from build123d import *

# Parameters (mm, degrees)
SKETCH1_R           = 6
BOSS_EXTRUDE1_DEPTH = 6.35
SKETCH2_W           = 6.35
SKETCH2_H           = 38.1
SKETCH2_W_2         = 31.75
SKETCH2_H_2         = 6.35
MOTORMOUNT_DEPTH    = 38.1
SKETCH4_W           = 6.35
SKETCH4_H           = 25.4
WHEELMOUNTS_DEPTH   = 38.1
FILLET1_R           = 6.35
BOSS_EXTRUDE4_START = -2.54
SKETCH5_R           = 6
SKETCH5_R_2         = 4.5
BOSS_EXTRUDE4_DEPTH = 2.54
SKETCH6_R           = 6
CUT_EXTRUDE2_DEPTH  = 83.947
FILLET2_R           = 6.35


with BuildPart() as part:
    # Sketch1 → Boss-Extrude1 (new body)
    with BuildSketch(Plane(origin=(0, 0, 0), x_dir=(1, 0, 0), z_dir=(0, 1, 0))):
        with BuildLine():
            Line((50.8, 0), (50.8, -28.575))
            Line((50.8, -28.575), (39.852082176, -33.3375))
            ThreePointArc((39.852082176, -33.3375), (33.608374366, -42.8625), (39.852082176, -52.3875))
            Line((39.852082176, -52.3875), (50.8, -57.15))
            Line((50.8, -57.15), (82.55, -57.15))
            Line((82.55, -57.15), (93.497917824, -52.3875))
            ThreePointArc((93.497917824, -52.3875), (99.741625634, -42.8625), (93.497917824, -33.3375))
            Line((93.497917824, -33.3375), (82.55, -28.575))
            Line((82.55, -28.575), (82.55, 0))
            Line((82.55, 0), (133.35, 0))
            Line((133.35, 0), (133.35, 95.25))
            Line((133.35, 95.25), (104.775, 95.25))
            Line((104.775, 95.25), (104.775, 142.875))
            Line((104.775, 142.875), (28.575, 142.875))
            Line((28.575, 142.875), (28.575, 95.25))
            Line((28.575, 95.25), (0, 95.25))
            Line((0, 95.25), (0, 0))
            Line((0, 0), (50.8, 0))
        make_face()
        with Locations(Location((89.354407321, -42.8625, 0), (0, 0, 270))):
            Circle(SKETCH1_R, mode=Mode.SUBTRACT)
        with Locations(Location((43.995592679, -42.8625, 0), (0, 0, 90))):
            Circle(SKETCH1_R, mode=Mode.SUBTRACT)
    extrude(amount=BOSS_EXTRUDE1_DEPTH)

    # Sketch2 → MotorMount (add)
    with BuildSketch(Plane(origin=(0, 6.35, 0), x_dir=(1, 0, 0), z_dir=(0, 1, 0))):
        with Locations((130.175, 76.2)):
            Rectangle(SKETCH2_W, SKETCH2_H)
        with Locations((3.175, 76.2)):
            Rectangle(SKETCH2_W, SKETCH2_H)
        with Locations((15.875, 3.175)):
            Rectangle(SKETCH2_W_2, SKETCH2_H_2)
        with Locations((117.475, 3.175)):
            Rectangle(SKETCH2_W_2, SKETCH2_H_2)
    extrude(amount=MOTORMOUNT_DEPTH)

    # Sketch4 → WheelMounts (add)
    with BuildSketch(Plane(origin=(0, 6.35, 0), x_dir=(1, 0, 0), z_dir=(0, 1, 0))):
        with Locations((101.6, 130.175)):
            Rectangle(SKETCH4_W, SKETCH4_H)
        with Locations((31.75, 130.175)):
            Rectangle(SKETCH4_W, SKETCH4_H)
    extrude(amount=WHEELMOUNTS_DEPTH)

    # Fillet1
    fillet1_edges = [part.edges().sort_by_distance(p)[0] for p in [
        (82.55, 3.175, 0),
        (50.8, 3.175, 0),
    ]]
    fillet(fillet1_edges, radius=FILLET1_R)

    # Sketch5 → Boss-Extrude4 (add)
    # profile 1 of 2: a face of its own
    with BuildSketch(Plane(origin=(0, 6.35, 0), x_dir=(1, 0, 0), z_dir=(0, 1, 0)).offset(BOSS_EXTRUDE4_START)):
        with Locations(Location((43.995592679, -42.8625, 0), (0, 0, 90))):
            Circle(SKETCH5_R)
        with Locations(Location((43.995592679, -42.8625, 0), (0, 0, 270))):
            Circle(SKETCH5_R_2, mode=Mode.SUBTRACT)
    # profile 2 of 2: a face of its own
    with BuildSketch(Plane(origin=(0, 6.35, 0), x_dir=(1, 0, 0), z_dir=(0, 1, 0)).offset(BOSS_EXTRUDE4_START)):
        with Locations(Location((89.354407321, -42.8625, 0), (0, 0, 270))):
            Circle(SKETCH5_R)
        with Locations(Location((89.354407321, -42.8625, 0), (0, 0, 270))):
            Circle(SKETCH5_R_2, mode=Mode.SUBTRACT)
    extrude(amount=BOSS_EXTRUDE4_DEPTH)

    # Sketch6 → Cut-Extrude2 (cut)
    with BuildSketch(Plane(origin=(104.775, 0, 0), x_dir=(0, 0, -1), z_dir=(1, 0, 0))):
        with Locations((132.715, 12.35)):
            Circle(SKETCH6_R)
    extrude(amount=-CUT_EXTRUDE2_DEPTH, mode=Mode.SUBTRACT)

    # Fillet2
    fillet2_edges = [part.edges().sort_by_distance(p)[0] for p in [
        (28.575, 3.175, -95.25),
        (104.775, 3.175, -95.25),
    ]]
    fillet(fillet2_edges, radius=FILLET2_R)


solid = part.part
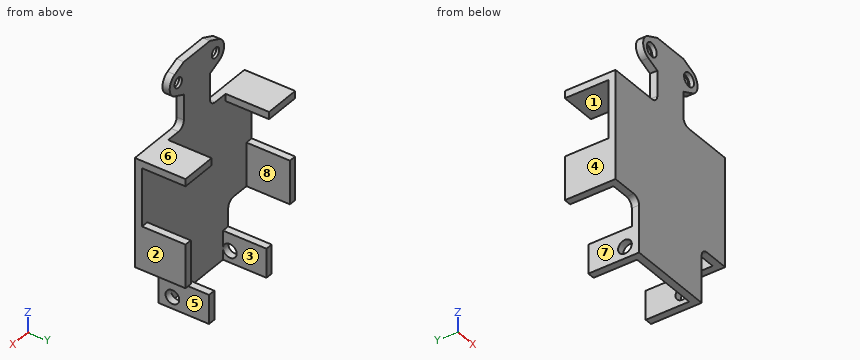
Geometry check sheet. Reference: the model listing, model coordinates, mm. Face numbers are marked on the shaded views. A direction names the side the tool comes from. Coordinates: 2 decimals unless noted, no trailing zeros. Loops run counter-clockwise (first coordinate to the right, second up) from the corner with the lowest first, then second, coordinate; pieces in that order, holes last. Notation, with made-up numbers: (-3.75, 88) - (16.25, 88) arc R19 cw to (16.25, 112) - close; hole circle Ø5 at (51.25, 78.5). An arc over 180 degrees is marked (long way). Use one line per item in the form item = value. Start each with the question number.
Item 1: Gauge pin test, flat ends, axial feed: pin 1 (6 mm diameter, centred on y = 25, z = -79, fed in from -X); pin 2 (13.5 mm diameter, centred on x = 113, y = 20, fed in from +Z); pin 3 (11 mm diameter, centred on y = 12.35, z = -132.715, fed in from -X); pin 4 (6 mm diameter, centred on x = 104, z = -29.5, fed in from +Y). Record the tip position at first contact, or that the pin passes through.
Item 2: Thickness scan on probe 1 along Z at (x, y) = (102, 12) (3 decimals); probe 2 along Z at (x, y) = (33, 12) (3 decimals); probe 3 along X at (y, z) = (26, -68). Record the ranges inside material, lowest first.
Item 3: Section check C-C, the plane z = -124. Enter the section's corners in (x, y) (3 decimals).
Item 4: Section check A-A, the plane y = 37. Enter the section's corners in (x, z) (3 decimals), and give its area (3 significant figures).
Item 5: Tool access check on the marked faces 1, 2, 3, 4 and 5. Record the directions out of +Z, -Z, +X, -X, +Y, -Y that give a thin tool (end or side, any length) a straight path to the whole face; none if there is none.
Item 6: Section check B-B, the plane y = 12.35. Give the number of separate pieces and of enclosed holes in the cut face, and give its area (3 significant figures).
Item 7: Section check D-D, the plane x = 15. Enter the section's corners in (y, z).
Item 8: Mould release check, pull along X, two halves, no side actions. Record for the marked faces 6, 7 and 8: +X half, -X half, draft (parallel to the pull), parting line (faces both ways), or undercut.
Computed:
q1.pin_1 = 0
q1.pin_2 = 0
q1.pin_3 = through
q1.pin_4 = 6.35
q2.probe_1 = -142.875 to -138.705, -126.725 to -117.475, -6.35 to 0
q2.probe_2 = -142.875 to -138.705, -126.725 to -117.475
q2.probe_3 = 0 to 6.35, 127 to 133.35
q3.outline = (28.575, 0) - (104.775, 0) - (104.775, 44.45) - (98.425, 44.45) - (98.425, 6.35) - (34.925, 6.35) - (34.925, 44.45) - (28.575, 44.45) - close
q4.outline = (0, -95.25) - (6.35, -95.25) - (6.35, -57.15) - (0, -57.15) - close; (0, -6.35) - (31.75, -6.35) - (31.75, 0) - (0, 0) - close; (28.575, -142.875) - (34.925, -142.875) - (34.925, -117.475) - (28.575, -117.475) - close; (98.425, -142.875) - (104.775, -142.875) - (104.775, -117.475) - (98.425, -117.475) - close; (101.6, -6.35) - (133.35, -6.35) - (133.35, 0) - (101.6, 0) - close; (127, -95.25) - (133.35, -95.25) - (133.35, -57.15) - (127, -57.15) - close
q4.area = 1,210 mm2
q5.face_1 = +X, -X, +Y
q5.face_2 = +Z, -Z, +X, +Y, -Y
q5.face_3 = +Z, -Z, +Y
q5.face_4 = +Z, -Z, -X, +Y, -Y
q5.face_5 = -Z, +X, +Y, -Y
q6.separate_pieces = 8
q6.enclosed_holes = 0
q6.area = 1,060 mm2
q7.outline = (0, -95.25) - (6.35, -95.25) - (6.35, -6.35) - (44.45, -6.35) - (44.45, 0) - (0, 0) - close
q8.face_6 = draft
q8.face_7 = -X half
q8.face_8 = undercut
